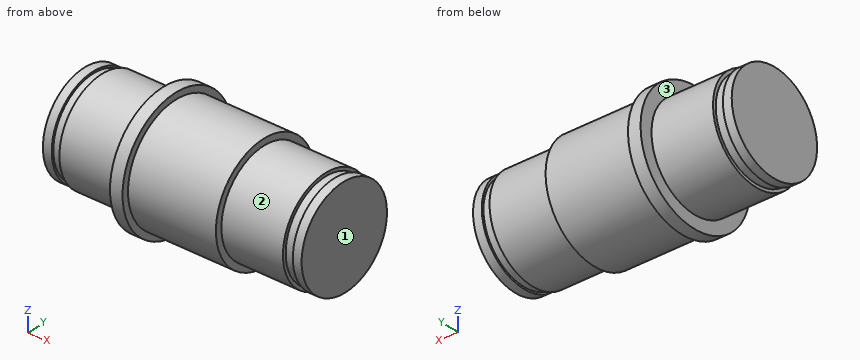
from build123d import *

# Parameters (mm, degrees)
SKETCH3_W = 1
SKETCH3_H = 0.5


with BuildPart() as part:
    # Sketch1 → Revolve1 (revolve)
    with BuildSketch(Plane.XY):
        Polygon((10.3, 0), (-10.3, 0), (-10.3, 3.9), (-9.6, 3.9), (-9.6, 3.75), (-8.9, 3.75), (-8.9, 4), (-4, 4), (-4, 4.5), (4, 4.5), (4, 4), (8.9, 4), (8.9, 3.75), (9.6, 3.75), (9.6, 3.9), (10.3, 3.9), align=None)
    revolve(axis=Axis((15.691805076, 0, 0), (-1, 0, 0)))

    # Sketch3 → Revolve2 (revolve)
    with BuildSketch(Plane.XY):
        with Locations((-3.5, 4.75)):
            Rectangle(SKETCH3_W, SKETCH3_H)
    revolve(axis=Axis((0, 0, 0), (-1, 0, 0)))


solid = part.part
Source: CAD feature listing. Evaluate the final solid. Frame: model axes, mm. Face numbers are marked on the shaded views. A direction names the side the tool comes from. Round coordinates to 2 decimals unless told otherwise and drop trailing zeros. Loops run counter-clockwise (first coordinate to the right, second up) from the corner with the lowest first, then second, coordinate; pieces in that order, holes last. Notation, with made-up numbers: (23, -29.75) - (52, -29.75) arc R29 cw to (52, 6.25) - close; hole circle Ø6 at (44, 5.25). An arc over 180 degrees is marked (long way). Write item = value, one per line. Start each with the question number.
Item 1: Section query C-C on x = 3. Output: boundary loops of the cut face in (y, z).
Item 2: First-contact query: pin 1 Ø6 at (x, y) = (8, -0.5) entering from -Z; pin 2 Ø1.5 at (x, z) = (7, -3.5) entering from +Y; pin 3 Ø1.5 at (x, y) = (2.5, 1.5) entering from -Z. Flat tips, straight axial feed; report the tip coordinate or a pass-through.
Item 3: Section query D-D on x = -7.75. Output: boundary loops of the cut face in (y, z).
Item 4: Material intervals for line 1 (X direction, y = -4, z = -2.5); line 2 (Y direction, x = -3.75, z = 3), sorted ascending.
Item 5: Reachability of the marked faces 1, 2 and 3 from +Z, -Z, +X, -X, +Y, -Y: full face, straight path, thin tool, end or side. Return the list, or none.
Results list:
q1.outline = circle Ø9 at (0, 0)
q2.pin_1 = -4
q2.pin_2 = 2.9
q2.pin_3 = -4.44
q3.outline = circle Ø8 at (0, 0)
q4.line_1 = -4 to -3
q4.line_2 = -4 to 4
q5.face_1 = +Z, -Z, +X, +Y, -Y
q5.face_2 = +X
q5.face_3 = -X
